Here's how the part is built. I have some questions about the finished solid (model axes, mm). A direction names the side the tool comes from. Coordinates: 2 decimals unless noted, no trailing zeros. Write each loop counter-clockwise with the first axis right and the second up, starting at its lowest first coordinate (ties: lowest second). Pieces come first, ordered by that corner, then holes.
(1) Imagine slicing it at B-B, the plane z = 2.15. List the corners of the cut face in (x, y) for me.
(2) Please list where these lines run through material, in increasing order: probe 1 along X at (y, z) = (6, 2.15); probe 2 along X at (y, z) = (-15.5, 1.05); probe 3 along Y at (x, z) = (136, 1.65).
(3) Imagine slicing it at A-A, the plane y = 4. List the corners of the cut face in (x, z) for me, plus the area to 3 significant figures.
(4) Which directions (+Z, -Z, +X, -X, +Y, -Y) give clear straight access to the entire face, cutting with the end or side of a thin tool? Please do faces 4 (the flat face through (149, -16, 1.25)), 5 (the flat face through (19.2, -1, 2)), 6 (the flat face through (15.2, -1, 3)).
(5) Thinking about a two-plate mould opening in Y: for faces 1 (the flat face through (149, -16, 3.75)), 2 (the flat face through (-3, 0, 2)), 3 (the flat face through (95, -14.95, 2)), which applies, released by +Y, released by -Y, zero draft, split by the parting line, or undercut?
(6) For pin 1 Ø2.5 at (x, z) = (7.5, 1.5) entering from -Y; pin 2 Ø1.5 at (y, z) = (1, 3) entering from +X; pin 3 Ø1.5 at (x, z) = (-3, 1.5) entering from -Y, each with a flat end and sliding along its axis, tell me the tip position at first contact or that it passes through.
(7) Imagine slicing it at C-C, the plane x = 43.5. List the corners of the cut face in (y, z) for me.
```python
from build123d import *

# Parameters (mm, degrees)
BOSS_EXTRUDE1_DEPTH = 5
SKETCH2_W           = 2.5
SKETCH2_H           = 2.5
BOSS_EXTRUDE2_DEPTH = 5
SKETCH3_W           = 3
SKETCH3_H           = 3
CUT_EXTRUDE1_DEPTH  = 10
SKETCH4_W           = 132.3
SKETCH4_H           = 1.5
CUT_EXTRUDE2_DEPTH  = 2
SKETCH5_W           = 3
SKETCH5_H           = 3
CUT_EXTRUDE3_DEPTH  = 12


with BuildPart() as part:
    # Sketch1 → Boss-Extrude1 (new body)
    with BuildSketch(Plane.XY):
        Polygon((0, 6.7), (0, 8.05), (5.5, 8.05), (14.2, 8.05), (14.2, -18.95), (146.5, -18.95), (146.5, -13.95), (19.2, -13.95), (19.2, 12.9), (5.5, 12.9), (-5, 12.9), (-5, 0), (0, 0), align=None)
    extrude(amount=BOSS_EXTRUDE1_DEPTH)

    # Sketch2 → Boss-Extrude2 (add)
    with BuildSketch(Plane(origin=(146.5, 0, 0), x_dir=(0, 0, -1), z_dir=(1, 0, 0))):
        with Locations((-2.5, -16.45)):
            Rectangle(SKETCH2_W, SKETCH2_H)
    extrude(amount=BOSS_EXTRUDE2_DEPTH)

    # Sketch3 → Cut-Extrude1 (cut)
    with BuildSketch(Plane.XY.offset(5)):
        with Locations((16.7, -0.6)):
            Rectangle(SKETCH3_W, SKETCH3_H)
    extrude(amount=-CUT_EXTRUDE1_DEPTH, mode=Mode.SUBTRACT)

    # Sketch4 → Cut-Extrude2 (cut)
    with BuildSketch(Plane.XY.offset(5)):
        with Locations((80.35, -16.45)):
            Rectangle(SKETCH4_W, SKETCH4_H)
    extrude(amount=-CUT_EXTRUDE2_DEPTH, mode=Mode.SUBTRACT)

    # Sketch5 → Cut-Extrude3 (cut)
    with BuildSketch(Plane(origin=(0, 0, 0), x_dir=(-1, 0, 0), z_dir=(0, 0, -1))):
        with Locations((-25.7, -16.45)):
            Rectangle(SKETCH5_W, SKETCH5_H)
        with Locations((-95, -16.45)):
            Rectangle(SKETCH5_W, SKETCH5_H)
    extrude(amount=-CUT_EXTRUDE3_DEPTH, mode=Mode.SUBTRACT)


solid = part.part
```
Recorded:
1. outline: (-5, 0) - (0, 0) - (0, 8.05) - (14.2, 8.05) - (14.2, -18.95) - (146.5, -18.95) - (146.5, -17.7) - (151.5, -17.7) - (151.5, -15.2) - (146.5, -15.2) - (146.5, -13.95) - (19.2, -13.95) - (19.2, 12.9) - (-5, 12.9) - close; hole (15.2, -2.1) - (18.2, -2.1) - (18.2, 0.9) - (15.2, 0.9) - close; hole (24.2, -17.95) - (27.2, -17.95) - (27.2, -14.95) - (24.2, -14.95) - close; hole (93.5, -17.95) - (96.5, -17.95) - (96.5, -14.95) - (93.5, -14.95) - close
2. probe 1: x = -5 to 0, 14.2 to 19.2
2. probe 2: x = 14.2 to 24.2, 27.2 to 93.5, 96.5 to 146.5
2. probe 3: y = -18.95 to -13.95
3. outline: (-5, 0) - (0, 0) - (0, 5) - (-5, 5) - close; (14.2, 0) - (19.2, 0) - (19.2, 5) - (14.2, 5) - close
3. area: 50.0 mm2
4. face 4: -Z, +X, +Y, -Y
4. face 5: +Z, -Z, +X, +Y
4. face 6: +Z, -Z
5. face 1: zero draft
5. face 2: released by -Y
5. face 3: undercut
6. pin 1: stops at y = 8.05
6. pin 2: stops at x = 19.2
6. pin 3: stops at y = 0
7. outline: (-18.95, 0) - (-13.95, 0) - (-13.95, 5) - (-15.7, 5) - (-15.7, 3) - (-17.2, 3) - (-17.2, 5) - (-18.95, 5) - close
